```python
from build123d import *

# Parameters (mm, degrees)
SKETCH1_W            = 18
SKETCH1_H            = 18
BOSS_EXTRUDE1_DEPTH  = 15
SKETCH3_R            = 5.306691295
CUT_EXTRUDE1_DEPTH   = 11.5
SKETCH4_W            = 18
SKETCH4_H            = 1.5
BOSS_EXTRUDE2_DEPTH  = 8
SKETCH6_W            = 18
SKETCH6_H            = 0.997263539
BOSS_EXTRUDE3_DEPTH  = 1
CUT_EXTRUDE2_DEPTH   = 18
SKETCH9_W            = 18
SKETCH9_H            = 1.5
BOSS_EXTRUDE4_DEPTH  = 1.5
SKETCH10_W           = 18
SKETCH10_H           = 1.5
BOSS_EXTRUDE6_DEPTH  = 3.25
SKETCH11_W           = 18
SKETCH11_H           = 1.625
BOSS_EXTRUDE7_DEPTH  = 1.5
SKETCH13_W           = 19.5
SKETCH13_H           = 1.5
BOSS_EXTRUDE9_DEPTH  = 1.5
SKETCH14_W           = 1.5
SKETCH14_H           = 19.5
BOSS_EXTRUDE10_DEPTH = 3.25
SKETCH15_W           = 19.5
SKETCH15_H           = 1.756529455
BOSS_EXTRUDE11_DEPTH = 1.5
SKETCH16_W           = 6
SKETCH16_H           = 1.5
BOSS_EXTRUDE12_DEPTH = 1.5
SKETCH17_W           = 1.5
SKETCH17_H           = 6
BOSS_EXTRUDE13_DEPTH = 3.25
SKETCH18_W           = 3
SKETCH18_H           = 1.625
BOSS_EXTRUDE14_DEPTH = 1.5
CUT_EXTRUDE3_DEPTH   = 18
CUT_EXTRUDE11_DEPTH  = 21
CUT_EXTRUDE12_DEPTH  = 2
CUT_EXTRUDE13_DEPTH  = 2


with BuildPart() as part:
    # Sketch1 → Boss-Extrude1 (new body)
    with BuildSketch(Plane(origin=(0, 0, 0), x_dir=(1, 0, 0), z_dir=(0, 1, 0))):
        with Locations((-5.757576823, 3.532227937)):
            Rectangle(SKETCH1_W, SKETCH1_H)
    extrude(amount=BOSS_EXTRUDE1_DEPTH)

    # Sketch3 → Cut-Extrude1 (cut)
    with BuildSketch(Plane(origin=(0, 15, 0), x_dir=(1, 0, 0), z_dir=(0, 1, 0))):
        with Locations((-5.757576823, 3.532227937)):
            Circle(SKETCH3_R)
    extrude(amount=-CUT_EXTRUDE1_DEPTH, mode=Mode.SUBTRACT)

    # Sketch4 → Boss-Extrude2 (add)
    with BuildSketch(Plane(origin=(0, 15, 0), x_dir=(1, 0, 0), z_dir=(0, 1, 0))):
        with Locations((-5.757576823, 11.782227937)):
            Rectangle(SKETCH4_W, SKETCH4_H)
    extrude(amount=BOSS_EXTRUDE2_DEPTH)

    # Sketch6 → Boss-Extrude3 (add)
    with BuildSketch(Plane.XY.offset(-11.032227937)):
        with Locations((-5.757576823, 22.50136823)):
            Rectangle(SKETCH6_W, SKETCH6_H)
    extrude(amount=BOSS_EXTRUDE3_DEPTH)

    # Sketch7 → Cut-Extrude2 (cut)
    with BuildSketch(Plane.ZY.offset(14.757576823)):
        Polygon((-11.032227937, 22.002736461), (-10.032227937, 23), (-10.032227937, 22.002736461), align=None)
    extrude(amount=-CUT_EXTRUDE2_DEPTH, mode=Mode.SUBTRACT)

    # Sketch9 → Boss-Extrude4 (add)
    with BuildSketch(Plane.XY.offset(5.467772063)):
        with Locations((-5.757576823, 0.75)):
            Rectangle(SKETCH9_W, SKETCH9_H)
    extrude(amount=BOSS_EXTRUDE4_DEPTH)

    # Sketch10 → Boss-Extrude6 (add)
    with BuildSketch(Plane.XZ):
        with Locations((-5.757576823, 6.217772063)):
            Rectangle(SKETCH10_W, SKETCH10_H)
    extrude(amount=BOSS_EXTRUDE6_DEPTH)

    # Sketch11 → Boss-Extrude7 (add)
    with BuildSketch(Plane(origin=(0, 0, 5.467772063), x_dir=(-1, 0, 0), z_dir=(0, 0, -1))):
        with Locations((5.757576823, -2.4375)):
            Rectangle(SKETCH11_W, SKETCH11_H)
    extrude(amount=BOSS_EXTRUDE7_DEPTH)

    # Sketch13 → Boss-Extrude9 (add)
    with BuildSketch(Plane.ZY.offset(14.757576823)):
        with Locations((-2.782227937, 0.75)):
            Rectangle(SKETCH13_W, SKETCH13_H)
    extrude(amount=BOSS_EXTRUDE9_DEPTH)

    # Sketch14 → Boss-Extrude10 (add)
    with BuildSketch(Plane.XZ):
        with Locations((-15.507576823, -2.782227937)):
            Rectangle(SKETCH14_W, SKETCH14_H)
    extrude(amount=BOSS_EXTRUDE10_DEPTH)

    # Sketch15 → Boss-Extrude11 (add)
    with BuildSketch(Plane(origin=(-14.757576823, 0, 0), x_dir=(0, 0, -1), z_dir=(1, 0, 0))):
        with Locations((2.782227937, -2.371735273)):
            Rectangle(SKETCH15_W, SKETCH15_H)
    extrude(amount=BOSS_EXTRUDE11_DEPTH)

    # Sketch16 → Boss-Extrude12 (add)
    with BuildSketch(Plane(origin=(3.242423177, 0, 0), x_dir=(0, 0, -1), z_dir=(1, 0, 0))):
        with Locations((-3.967772063, 0.75)):
            Rectangle(SKETCH16_W, SKETCH16_H)
    extrude(amount=BOSS_EXTRUDE12_DEPTH)

    # Sketch17 → Boss-Extrude13 (add)
    with BuildSketch(Plane.XZ):
        with Locations((3.992423177, 3.967772063)):
            Rectangle(SKETCH17_W, SKETCH17_H)
    extrude(amount=BOSS_EXTRUDE13_DEPTH)

    # Sketch18 → Boss-Extrude14 (add)
    with BuildSketch(Plane.ZY.offset(-3.242423177)):
        with Locations((2.467772063, -2.4375)):
            Rectangle(SKETCH18_W, SKETCH18_H)
    extrude(amount=BOSS_EXTRUDE14_DEPTH)

    # Sketch19 → Cut-Extrude3 (cut)
    with BuildSketch(Plane(origin=(0, 0, -12.532227937), x_dir=(-1, 0, 0), z_dir=(0, 0, -1))):
        Polygon((16.257576823, 0), (14.757576823, 1.5), (16.257576823, 1.5), align=None)
        Polygon((-4.742423177, 0), (-3.242423177, 1.5), (-4.742423177, 1.5), align=None)
    extrude(amount=-CUT_EXTRUDE3_DEPTH, mode=Mode.SUBTRACT)

    # Sketch22 → Cut-Extrude11 (cut)
    with BuildSketch(Plane(origin=(4.742423177, 0, 0), x_dir=(0, 0, -1), z_dir=(1, 0, 0))):
        Polygon((-6.967772063, 0), (-6.967772063, 1.5), (-5.467772063, 1.5), align=None)
    extrude(amount=-CUT_EXTRUDE11_DEPTH, mode=Mode.SUBTRACT)

    # Sketch24 → Cut-Extrude12 (cut)
    with BuildSketch(Plane(origin=(0, 0, 5.467772063), x_dir=(-1, 0, 0), z_dir=(0, 0, -1))):
        Polygon((-3.242423177, 1.5), (-4.742423177, 0), (-4.742423177, 1.5), align=None)
    extrude(amount=-CUT_EXTRUDE12_DEPTH, mode=Mode.SUBTRACT)

    # Sketch25 → Cut-Extrude13 (cut)
    with BuildSketch(Plane(origin=(0, 0, 5.467772063), x_dir=(-1, 0, 0), z_dir=(0, 0, -1))):
        Polygon((16.257576823, 0), (14.757576823, 1.5), (16.257576823, 1.5), align=None)
    extrude(amount=-CUT_EXTRUDE13_DEPTH, mode=Mode.SUBTRACT)


solid = part.part
```
Source: CAD feature listing. Evaluate the final solid. Frame: model axes, mm. A direction names the side the tool comes from. Round coordinates to 2 decimals unless told otherwise and drop trailing zeros. Loops run counter-clockwise (first coordinate to the right, second up) from the corner with the lowest first, then second, coordinate; pieces in that order, holes last.
(1) Section query B-B (x = -11.5). Output: boundary loops of the cut face in (y, z) (3 decimals), and give its area (3 significant figures).
From the geometry:
outline: (-3.25, 3.968) - (-1.625, 3.968) - (-1.625, 5.468) - (0, 5.468) - (0, -12.532) - (23, -12.532) - (23, -10.032) - (22.003, -11.032) - (15, -11.032) - (15, 5.468) - (1.5, 5.468) - (0, 6.968) - (-3.25, 6.968) - close
area: 291 mm2
(2) Material intervals for probe 1 along Y at (x, z) = (-2.5, -3.25); probe 2 along X at (y, z) = (-1, -0.25); probe 3 along Z at (x, y) = (-7.25, 1.5), sorted ascending.
From the geometry:
probe 1: y = 0 to 3.5
probe 2: x = -16.26 to -14.76
probe 3: z = -12.53 to 5.47
(3) Section query D-D (y = 18.75). Output: boundary loops of the cut face in (x, z), and give its area (3 significant figures).
From the geometry:
outline: (-14.76, -12.53) - (3.24, -12.53) - (3.24, -11.03) - (-14.76, -11.03) - close
area: 27.0 mm2
(4) Access query for faces 4 (the flat face through (1.742, -2, 2)), 5 (the flat face through (4, -1, 0.968)), 6 (the flat face through (-6, 18, -11.032)). Directions: +Z, -Z, +X, -X, +Y, -Y. A direction counts if a zero-diameter tool reaches every point of the face in a straight line with its end or side. Return the directions, or none.
From the geometry:
face 4: -Z, -Y
face 5: -Z, +X, -Y
face 6: +Z, +X, -X
(5) Contact query for flat-ended pins moving along their axis: pin 1 Ø2 at (x, z) = (-3.5, 4) entering from +Y; pin 2 Ø6 at (x, z) = (-0.5, -2.5) entering from -Y; pin 3 Ø9 at (y, z) = (10.5, -6) entering from +X. Output: stop coordinate, or through.
From the geometry:
pin 1: stops at y = 15
pin 2: stops at y = 0
pin 3: stops at x = 3.24
(6) Section query C-C (z = -9.5). Output: boundary loops of the cut face in (x, y).
From the geometry:
outline: (-16.26, -3.25) - (-13.26, -3.25) - (-13.26, -1.49) - (-14.76, -1.49) - (-14.76, 0) - (3.24, 0) - (3.24, 15) - (-14.76, 15) - (-14.76, 1.5) - (-16.26, 0) - close
(7) Section query A-A (z = 5). Output: boundary loops of the cut face in (x, y) (3 decimals).
From the geometry:
outline: (-16.258, -3.25) - (4.742, -3.25) - (4.742, 0) - (3.242, 1.5) - (3.242, 15) - (-14.758, 15) - (-14.758, 1.5) - (-16.258, 0) - close; hole (-14.758, -1.493) - (-13.258, -1.493) - (-13.258, -1.625) - (3.242, -1.625) - (3.242, 0) - (-14.758, 0) - close
(8) Pull-direction query (Y, two-part tool) for faces 1 (the flat face through (-15.52, 0.74, -2.92)), 2 (the flat face through (-6, 0, -3)), 3 (the flat face through (-7, 10, -12.532)); classes: +Y half, -Y half, draft (parallel to the pull), parting line (faces both ways), or undercut.
From the geometry:
face 1: +Y half
face 2: undercut
face 3: draft
